Here's how the part is built. I have some questions about the finished solid (model axes, mm). Round coordinates to 2 decimals unless told otherwise and drop trailing zeros. Write each loop counter-clockwise with the first axis right and the second up, starting at its lowest first coordinate (ties: lowest second). Pieces come first, ordered by that corner, then holes. Notation, with made-up numbers: M -34,10 L 19,10 A23 ccw 19,34 Z; hole C -24,25.5 d4. An arc over 180 degrees is marked long. Write item = value, one per line. Start each with the question number.
(1) I need wall thicknesses on line 1 along X through (y, z) = (532, 436); line 2 along Z through (x, y) = (316, 798.5); line 3 along X through (y, z) = (561.5, 491). Which ranges of each line are inside material? Lowest first, please.
(2) I want a section at B-B (z = 432). List the corners of the cut face in (x, y) for me.
(3) I want a section at C-C (x = 318). List the corners of the cut face in (y, z) for me.
(4) I want a section at A-A (y = 581). List the corners of the cut face in (x, z) for me.
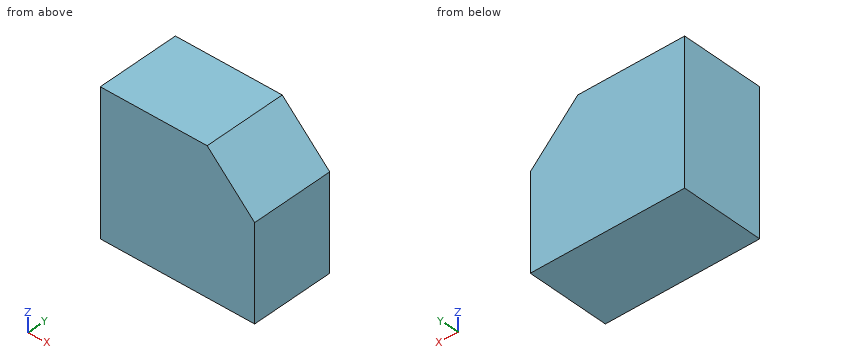
```python
from build123d import *

# Parameters (mm, degrees)
SKETCH_1_W          = 503
SKETCH_1_H          = 558
EXTRUDE_1_DEPTH     = 865
SKETCH_2_W          = 200
SKETCH_2_H          = 398
CUT_EXTRUDE_1_DEPTH = 1039.785348376
SKETCH_3_W          = 94
SKETCH_3_H          = 148
CUT_EXTRUDE_2_DEPTH = 1039.785348376
SKETCH_5_W          = 650
SKETCH_5_H          = 350
EXTRUDE_3_DEPTH     = 600
CHAMFER_1_SIZE      = 200
SKETCH_6_W          = 1000
SKETCH_6_H          = 4830
EXTRUDE_4_DEPTH     = 30
SKETCH_7_W          = 625.774769939
SKETCH_7_H          = 5017.85714808
CUT_EXTRUDE_3_DEPTH = 3931.092365327
SKETCH_8_W          = 1324.574856274
SKETCH_8_H          = 1226.736940753
CUT_EXTRUDE_4_DEPTH = 1300.413329161


with BuildPart() as part:
    # 草图1 → 凸台-拉伸1 (new body)
    with BuildSketch(Plane.XY):
        Rectangle(SKETCH_1_W, SKETCH_1_H)
    extrude(amount=EXTRUDE_1_DEPTH)

    # 草图2 → 切除-拉伸1 (cut, through all)
    with BuildSketch(Plane(origin=(251.5, 0, 0), x_dir=(0, 0, -1), z_dir=(1, 0, 0))):
        Rectangle(SKETCH_2_W, SKETCH_2_H)
    extrude(amount=-CUT_EXTRUDE_1_DEPTH, mode=Mode.SUBTRACT)

    # 草图3 → 切除-拉伸2 (cut, through all)
    with BuildSketch(Plane(origin=(251.5, 0, 0), x_dir=(0, 0, -1), z_dir=(1, 0, 0))):
        with Locations((-53, -279)):
            Rectangle(SKETCH_3_W, SKETCH_3_H)
    cut_extrude_2 = extrude(amount=-CUT_EXTRUDE_2_DEPTH, mode=Mode.SUBTRACT)

    # 镜向1: 切除-拉伸2 across plane
    add(cut_extrude_2.mirror(Plane.ZX), mode=Mode.SUBTRACT)

    # 草图8 → 切除-拉伸4 (cut, through all)
    with BuildSketch(Plane(origin=(251.5, 0, 0), x_dir=(0, 0, -1), z_dir=(1, 0, 0))):
        with Locations((-463.569646277, -264.855691223)):
            Rectangle(SKETCH_8_W, SKETCH_8_H)
    extrude(amount=-CUT_EXTRUDE_4_DEPTH, mode=Mode.SUBTRACT)


with BuildPart() as body_2:
    # 草图5 → 凸台-拉伸3 (new body)
    with BuildSketch(Plane(origin=(0, 0, 0), x_dir=(-1, 0, 0), z_dir=(0, 0, -1))):
        with Locations((-73.5, 654)):
            Rectangle(SKETCH_5_W, SKETCH_5_H)
    extrude(amount=-EXTRUDE_3_DEPTH)

    # 倒角1
    chamfer_1_edges = [body_2.edges().sort_by_distance(p)[0] for p in [
        (398.5, 654, 600),
    ]]
    chamfer(chamfer_1_edges, length=CHAMFER_1_SIZE)


with BuildPart() as body_3:
    # 草图6 → 凸台-拉伸4 (new body)
    with BuildSketch(Plane(origin=(0, 0, 0), x_dir=(-1, 0, 0), z_dir=(0, 0, -1))):
        with Locations((-248.5, -1286)):
            Rectangle(SKETCH_6_W, SKETCH_6_H)
    extrude(amount=EXTRUDE_4_DEPTH)

    # 草图7 → 切除-拉伸3 (cut, through all)
    with BuildSketch(Plane(origin=(748.5, 0, 0), x_dir=(0, 0, -1), z_dir=(1, 0, 0))):
        with Locations((312.88738497, -1379.92857404)):
            Rectangle(SKETCH_7_W, SKETCH_7_H)
    extrude(amount=-CUT_EXTRUDE_3_DEPTH, mode=Mode.SUBTRACT)


solid = body_2.part
```
Returned:
q1.line_1 = -251.5 to 362.5
q1.line_2 = 0 to 482.5
q1.line_3 = -251.5 to 307.5
q2.outline = M -251.5,479 L 366.5,479 L 366.5,829 L -251.5,829 Z
q3.outline = M 479,0 L 829,0 L 829,480.5 L 479,480.5 Z
q4.outline = M -251.5,0 L 398.5,0 L 398.5,400 L 198.5,600 L -251.5,600 Z
